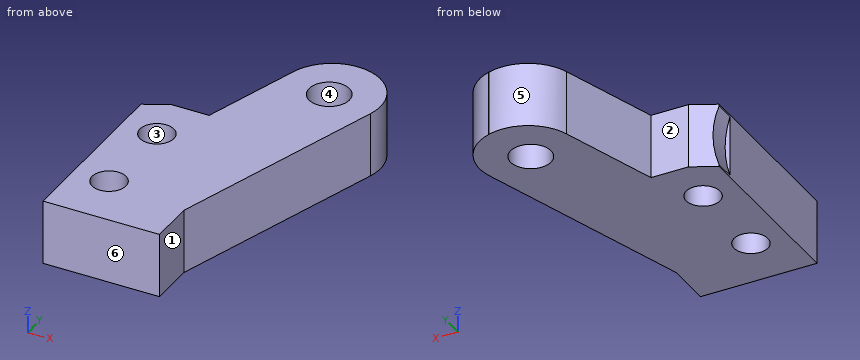
```python
from build123d import *

# Parameters (mm, degrees)
CYLINDER749_R          = 1.25
CYLINDER749_DEPTH      = 6
CYLINDER792_R          = 6.1
CYLINDER792_DEPTH      = 8
CYLINDER789_R          = 1.05
CYLINDER789_DEPTH      = 37
CYLINDER790_R          = 1.05
CYLINDER790_DEPTH      = 37
CYLINDER791_R          = 1.05
CYLINDER791_DEPTH      = 37
CYLINDER788_R          = 1.05
CYLINDER788_DEPTH      = 37
BOX289_W               = 7.2
BOX289_H               = 12
BOX289_DEPTH           = 4
BOX284_W               = 18
BOX284_H               = 6
BOX284_DEPTH           = 4
BOX284_PLACEMENT_ANGLE = 72.5
FILLET125007020021_R   = 2.99
CHAMFER228022_SIZE2    = 1.5
CHAMFER228022_SIZE     = 0.75


with BuildPart() as cylinder749:
    # Cylinder749 → Cylinder749 (new body)
    with BuildSketch(Plane(origin=(14.35, 41, -3), x_dir=(1, 0, 0), z_dir=(0, 0, 1))):
        Circle(CYLINDER749_R)
    extrude(amount=CYLINDER749_DEPTH)


with BuildPart() as cylinder792:
    # Cylinder792 → Cylinder792 (new body)
    with BuildSketch(Plane(origin=(0, 34, 0), x_dir=(1, 0, 0), z_dir=(0, 1, 0))):
        Circle(CYLINDER792_R)
    extrude(amount=CYLINDER792_DEPTH)


with BuildPart() as cylinder789:
    # Cylinder789 → Cylinder789 (new body)
    with BuildSketch(Plane(origin=(8, 33, -19), x_dir=(1, 0, 0), z_dir=(0, 0, 1))):
        Circle(CYLINDER789_R)
    extrude(amount=CYLINDER789_DEPTH)


with BuildPart() as cylinder790:
    # Cylinder790 → Cylinder790 (new body)
    with BuildSketch(Plane(origin=(-8, 33, -19), x_dir=(1, 0, 0), z_dir=(0, 0, 1))):
        Circle(CYLINDER790_R)
    extrude(amount=CYLINDER790_DEPTH)


with BuildPart() as cylinder791:
    # Cylinder791 → Cylinder791 (new body)
    with BuildSketch(Plane(origin=(8, 27.5, -19), x_dir=(1, 0, 0), z_dir=(0, 0, 1))):
        Circle(CYLINDER791_R)
    extrude(amount=CYLINDER791_DEPTH)


with BuildPart() as fusion088026007031024007008004081011:
    # Cylinder788 → Cylinder788 (new body)
    with BuildSketch(Plane(origin=(-8, 27.5, -19), x_dir=(1, 0, 0), z_dir=(0, 0, 1))):
        Circle(CYLINDER788_R)
    extrude(amount=CYLINDER788_DEPTH)

    # Fusion088026007031024007008004081011: union Cylinder789, Cylinder790, Cylinder791
    add(cylinder789.part)
    add(cylinder790.part)
    add(cylinder791.part)


with BuildPart() as cube288:
    # Box289 → Box289 (new body)
    with BuildSketch(Plane(origin=(5.8, 24, -2), x_dir=(1, 0, 0), z_dir=(0, 0, 1))):
        with Locations((3.6, 6)):
            Rectangle(BOX289_W, BOX289_H)
    extrude(amount=BOX289_DEPTH)


with BuildPart() as cut176013009033007019019008010045:
    # Box284 → Box284 (new body)
    with BuildSketch(Plane.XY):
        with Locations((9, 3)):
            Rectangle(BOX284_W, BOX284_H)
    extrude(amount=BOX284_DEPTH)


with BuildPart() as cut176013009033007019019008010045_1:
    # Box284 placement: moved
    add(cut176013009033007019019008010045.part.moved(Location((12.75, 26, -2))).rotate(Axis((12.75, 26, -2), (0, 0, 1)), BOX284_PLACEMENT_ANGLE))

    # Fillet125007020021
    fillet125007020021_edges = [cut176013009033007019019008010045_1.edges().sort_by_distance(p)[0] for p in [
        (18.162704, 43.166905, 0),
        (12.440403, 44.97114, 0),
    ]]
    fillet(fillet125007020021_edges, radius=FILLET125007020021_R)

    # Fusion088026007031024007008004081010: union Cube288
    add(cube288.part)

    # Cut176013009033007019019008010043: cut Fusion088026007031024007008004081011
    add(fusion088026007031024007008004081011.part, mode=Mode.SUBTRACT)

    # Chamfer228022
    chamfer228022_edges = [cut176013009033007019019008010045_1.edges().sort_by_distance(p)[0] for p in [
        (5.8, 36, 0),
    ]]
    chamfer228022_side = cut176013009033007019019008010045_1.faces().sort_by_distance((5.8, 30, 0))[0]
    chamfer(chamfer228022_edges, length=CHAMFER228022_SIZE, length2=CHAMFER228022_SIZE2, reference=chamfer228022_side)

    # Cut176013009033007019019008010044: cut Cylinder792
    add(cylinder792.part, mode=Mode.SUBTRACT)

    # Cut176013009033007019019008010045: cut Cylinder749
    add(cylinder749.part, mode=Mode.SUBTRACT)


with BuildPart() as cut176013009033007019019008010045_2:
    # Cut176013009033007019019008010045 placement: moved
    add(cut176013009033007019019008010045_1.part.moved(Location((75, -93, 46))))


solid = cut176013009033007019019008010045_2.part
```
Source: CAD feature listing. Evaluate the final solid. Frame: model axes, mm. Face numbers are marked on the shaded views. A direction names the side the tool comes from. Give positions to 0.01 mm unless a question says otherwise; leave off trailing zeros. Loops run counter-clockwise (first coordinate to the right, second up) from the corner with the lowest first, then second, coordinate; pieces in that order, holes last. Notation, with made-up numbers: (15.5, 44) - (32.5, 44) arc R7 cw to (32.5, 51) - close; hole circle Ø7 at (11.25, 57.5). An arc over 180 degrees is marked (long way). Use CSV: the item, a comma, the result in double quotes.
1) Cut plane B-B (x = 89.5). Output: boundary loops of the cut face in (y, z).
Worked out:
outline,"(-61.45, 44) - (-53.24, 44) - (-53.24, 48) - (-61.45, 48) - close; (-50.76, 44) - (-48.79, 44) - (-48.79, 48) - (-50.76, 48) - close"
2) Mould query, pull axis X, two halves, no side actions, for the marked faces 4, 5 and 6. Classes: +X half, -X half, draft (parallel to the pull), parting line (faces both ways), or undercut.
Worked out:
face 4,"undercut"
face 5,"parting line"
face 6,"draft"
3) Pin query (flat end, axial travel): P1, Ø2, axis at x = 89.35, y = -52, coming from the +Z side. Return the tip coordinate at first contact, or that it passes through.
Worked out:
P1,"passes through"
4) Cut plane C-C (y = -65.5). Output: boundary loops of the cut face in (x, z), and give its area (3 significant figures).
Worked out:
outline,"(80.8, 44) - (81.95, 44) - (81.95, 48) - (80.8, 48) - close; (84.05, 44) - (88.22, 44) - (88.22, 48) - (84.05, 48) - close"
area,"21.3 mm^2"
5) Set-up query: the marked faces 1, 2 and 3. Return all of +Z, -Z, +X, -X, +Y, -Y with unobstructed straight access to the full face (end or side cutting, diameter ignored); none if empty.
Worked out:
face 1,"+Z, -Z, +X, -Y"
face 2,"+Z, -Z, -X, +Y"
face 3,"+Z, -Z"
6) Cut plane A-A (z = 47.1). Count the separate pieces of the cut face and the enclosed holes in it, and give its area (3 significant figures).
Worked out:
separate pieces,"1"
enclosed holes,"3"
area,"134 mm^2"
7) Line query: line 1 (Y direction, x = 83, z = 45.35); line 2 (X direction, y = -65.5, z = 45.8); line 3 (X direction, y = -52, z = 45.05). Output: solid intervals per line, ascending.
Worked out:
line 1,"y = -69 to -66.55, -64.45 to -61.05, -58.95 to -57"
line 2,"x = 80.8 to 81.95, 84.05 to 88.22"
line 3,"x = 86.19 to 88.1, 90.6 to 92.39"
